Input: part model. Units: mm. Frame: model coordinates. Give positions to 0.01 mm unless a question says otherwise; leave off trailing zeros. Write each loop counter-clockwise with the first axis right and the second up, starting at its lowest first coordinate (ties: lowest second). Pieces come first, ordered by that corner, then holes. Notation, with made-up numbers: M 11,-1 L 55,-1 A24 ccw 55,33 Z; hole C 66,26 d6. An arc over 180 degrees is marked long. Use CSV: the item, a comma, the result in double quotes. Start each with the question number.
from build123d import *

# Parameters (mm, degrees)
F0_R     = 31.75
F1_DEPTH = 254
F2_R     = 5.08
F3_R     = 5.08
F4_R     = 12.7
F5_DEPTH = 254.001
F6_R     = 5.08


with BuildPart() as f1:
    # F0 (on Front) → F1 (new body)
    with BuildSketch(Plane.XZ):
        Circle(F0_R)
    extrude(amount=F1_DEPTH)

    # F2
    f2_edges = [f1.edges().sort_by_distance(p)[0] for p in [
        (-31.75, -254, 0),
    ]]
    fillet(f2_edges, radius=F2_R)

    # F3
    f3_edges = [f1.edges().sort_by_distance(p)[0] for p in [
        (-31.75, 0, 0),
    ]]
    fillet(f3_edges, radius=F3_R)

    # F4 (on face) → F5 (cut, through all)
    with BuildSketch(Plane(origin=(0, 0, 0), x_dir=(-1, 0, 0), z_dir=(0, 1, 0))):
        Circle(F4_R)
    extrude(amount=-F5_DEPTH, mode=Mode.SUBTRACT)

    # F6
    f6_edges = [f1.edges().sort_by_distance(p)[0] for p in [
        (12.7, 0, 0),
        (-12.7, -127, 0),
        (12.7, -254, 0),
    ]]
    fillet(f6_edges, radius=F6_R)


solid = f1.part
Q1. Material intervals for L1, parallel to Z at x = 0, y = -149.5; L2, parallel to X at y = -217, z = 0.5; L3, parallel to Z at x = 5.5, y = -202.5, sorted ascending. Write a range as [from, to].
Q2. Section C-C, the plane y = -138.5. Return the cut outline in (x, z).
Q3. Section B-B, the plane x = 0. Return the cut outline in (y, z), and give its area (3 significant figures).
Q4. First-contact query: pin 1 Ø1.5 at (y, z) = (-31, 9) entering from -X; pin 2 Ø3 at (y, z) = (-118, 19) entering from -X; pin 3 Ø5 at (x, y) = (24, -119) entering from +Z. Flat tips, straight axial feed; report the tip coordinate or a pass-through.
Q5. Pull-direction query (Z, two-part tool) for faces 1 (the flat face through (17, 0, -6)), 2 (the cylindrical face through (2.75, -125.29, -12.4)), 3 (the cylindrical face through (-6.883, -125.293, -30.995)); classes: released by +Z, released by -Z, zero draft, split by the parting line, or undercut.
Q6. Section A-A, the plane z = 0. Return the cut outline in (x, y).
Check result:
1,L1,"z = [-31.75, -12.7], [12.7, 31.75]"
1,L2,"x = [-31.75, -12.69], [12.69, 31.75]"
1,L3,"z = [-31.27, -11.45], [11.45, 31.27]"
2,outline,"C 0,0 d63.5; hole C 0,0 d25.4"
3,outline,"M -254,-26.67 A5.08 ccw -248.92,-31.75 L -5.08,-31.75 A5.08 ccw 0,-26.67 L 0,-17.78 A5.08 ccw -5.08,-12.7 L -248.92,-12.7 A5.08 ccw -254,-17.78 Z; M -254,17.78 A5.08 ccw -248.92,12.7 L -5.08,12.7 A5.08 ccw 0,17.78 L 0,26.67 A5.08 ccw -5.08,31.75 L -248.92,31.75 A5.08 ccw -254,26.67 Z"
3,area,"9,630 mm²"
4,pin 1,"stops at x = -30.66"
4,pin 2,"stops at x = -26.49"
4,pin 3,"stops at z = 23.36"
5,face 1,"zero draft"
5,face 2,"undercut"
5,face 3,"split by the parting line"
6,outline,"M -31.75,-248.92 A5.08 ccw -26.67,-254 L -17.78,-254 A5.08 ccw -12.7,-248.92 L -12.7,-5.08 A5.08 ccw -17.78,0 L -26.67,0 A5.08 ccw -31.75,-5.08 Z; M 12.7,-248.92 A5.08 ccw 17.78,-254 L 26.67,-254 A5.08 ccw 31.75,-248.92 L 31.75,-5.08 A5.08 ccw 26.67,0 L 17.78,0 A5.08 ccw 12.7,-5.08 Z"
